For this review, take the finished solid that the model builds, in its own axes (mm). Coordinates: 2 decimals unless noted, no trailing zeros. Write each loop counter-clockwise with the first axis right and the second up, starting at its lowest first coordinate (ties: lowest second). Pieces come first, ordered by that corner, then holes. Notation, with made-up numbers: (41.25, 78) - (56.25, 78) arc R25 ccw to (56.25, 99) - close; hole circle Ø6 at (28.5, 56). An arc over 180 degrees is marked (long way). Write each question's results on one line, items separated by ' | '.
from build123d import *

# Parameters (mm, degrees)
F1_DEPTH = 4


with BuildPart() as f1:
    # F0 (on Top) → F1 (new body)
    with BuildSketch(Plane.XY):
        Polygon((-20, 0), (0, 0), (0, 20), (-4, 20), (-4, 40), (0, 40), (0, 60), (-3.561152, 60), (-3.561152, 80), (0, 80), (0, 100), (-20, 100), (-20, 96), (-40, 96), (-40, 100), (-60, 100), (-60, 96), (-80, 96), (-80, 100), (-100, 100), (-100, 96), (-120, 96), (-120, 100), (-140, 100), (-140, 96), (-160, 96), (-160, 100), (-180, 100), (-180, 96), (-200, 96), (-200, 100), (-220, 100), (-220, 96), (-240, 96), (-240, 100), (-260, 100), (-260, 96), (-280, 96), (-280, 100), (-300, 100), (-300, 80), (-296, 80), (-296, 60), (-300, 60), (-300, 40), (-296, 40), (-296, 20), (-300, 20), (-300, 0), (-280, 0), (-280, 4), (-260, 4), (-260, 0), (-240, 0), (-240, 4), (-220, 4), (-220, 0), (-200, 0), (-200, 4), (-180, 4), (-180, 0), (-160, 0), (-160, 4), (-140, 4), (-140, 0), (-120, 0), (-120, 4), (-100, 4), (-100, 0), (-80, 0), (-80, 4), (-60, 4), (-60, 0), (-40, 0), (-40, 4), (-20, 4), align=None)
    extrude(amount=F1_DEPTH)


solid = f1.part
Q1. For pin 1 (1.2 mm diameter, centred on x = -193.5, z = 1, fed in from -Y); pin 2 (1 mm diameter, centred on y = 74, z = 3.5, fed in from -X), all flat-tipped, find the tip position at first contact; note any pin that passes through.
Results found:
pin 1: y = 4 | pin 2: x = -296
Q2. Take a section at A-A on y = 66. State the section outline as (x, z) points, plus the area to 3 significant figures.
Results found:
outline: (-296, 0) - (-3.56, 0) - (-3.56, 4) - (-296, 4) - close | area: 1,170 mm2
Q3. Wall thickness on line 1 along X through (y, z) = (37.5, 3.5); line 2 along Y through (x, z) = (-235, 0.8); line 3 along X through (y, z) = (78, 2.1): over which ranges is each line inside the solid? List them lowest first. Write a range as from..to.
Results found:
line 1: -296..-4 | line 2: 4..96 | line 3: -296..-3.56
Q4. Take a section at B-B on x = -226. State the section outline as (y, z) points, plus the area to 3 significant figures.
Results found:
outline: (4, 0) - (96, 0) - (96, 4) - (4, 4) - close | area: 368 mm2
